Part model, mm, in its own coordinate system. Round coordinates to 2 decimals unless told otherwise and drop trailing zeros. Loops run counter-clockwise (first coordinate to the right, second up) from the corner with the lowest first, then second, coordinate; pieces in that order, holes last.
(1) Mould opens along X. For faces 1 (the face through (-27.1, 3.04, 51.66)), 2 (the face through (28.9, 3.04, 51.66)), 3 (the face through (-1, 6, -2)), 4 (the face through (85, 3, 2)) say: +X half, -X half, draft (parallel to the pull), parting line (faces both ways), or undercut.
(2) Cut at C-C on x = -42.5. List the corners of the cut face in (y, z).
(3) Cut at B-B on y = 4. Count the separate pieces of the cut face and the enclosed holes in it, then the cut area to 3 significant figures.
(4) Flat gauge pin, fed straight in: pin 1 (8 mm diameter, centred on x = 0, z = -13.7, fed in from +Y). Where does the tip first touch, or does it go through?
(5) Probe probe 1 along X at (y, z) = (3.3, 48.8); probe 2 along X at (y, z) = (4, 92.5); probe 3 along X at (y, z) = (3.5, -124.5). List the from-to ranges inside material, lowest first.
(6) Cut at D-D on z = -13.7. List the corners of the cut face in (x, y), then the cut area to 3 significant figures.
(7) Cut at A-A on z = 92.5. List the corners of the cut face in (x, y).
from build123d import *

# Parameters (mm, degrees)
SKETCH1_W           = 170
SKETCH1_H           = 280
BOSS_EXTRUDE1_DEPTH = 6
SKETCH2_R           = 5
CUT_EXTRUDE1_DEPTH  = 6
SKETCH4_R           = 22.5
SKETCH4_R_2         = 3
CUT_EXTRUDE3_DEPTH  = 10


with BuildPart() as part:
    # Sketch1 → Boss-Extrude1 (new body)
    with BuildSketch(Plane(origin=(0, 0, 0), x_dir=(1, 0, 0), z_dir=(0, 1, 0))):
        Rectangle(SKETCH1_W, SKETCH1_H)
    extrude(amount=BOSS_EXTRUDE1_DEPTH)

    # Sketch2 → Cut-Extrude1 (cut)
    with BuildSketch(Plane(origin=(0, 6, 0), x_dir=(1, 0, 0), z_dir=(0, 1, 0))):
        with Locations(Location((-57.5, 120, 0), (0, 0, 270))):
            Circle(SKETCH2_R)
        with Locations(Location((57.5, 120, 0), (0, 0, 270))):
            Circle(SKETCH2_R)
        with Locations(Location((0, 13.7, 0), (0, 0, 270))):
            Circle(SKETCH2_R)
        with Locations(Location((-57.5, -120, 0), (0, 0, 270))):
            Circle(SKETCH2_R)
        with Locations(Location((57.5, -120, 0), (0, 0, 270))):
            Circle(SKETCH2_R)
        with Locations(Location((-42.5, -92.5, 0), (0, 0, 270))):
            Circle(SKETCH2_R)
        with Locations(Location((42.5, -92.5, 0), (0, 0, 270))):
            Circle(SKETCH2_R)
    extrude(amount=-CUT_EXTRUDE1_DEPTH, mode=Mode.SUBTRACT)

    # Sketch4 → Cut-Extrude3 (cut)
    with BuildSketch(Plane(origin=(0, 6, 0), x_dir=(1, 0, 0), z_dir=(0, 1, 0))):
        with Locations(Location((0, -48.8, 0), (0, 0, 270))):
            Circle(SKETCH4_R)
        with Locations(Location((28, -48.8, 0), (0, 0, 270))):
            Circle(SKETCH4_R_2)
        with Locations(Location((-28, -48.8, 0), (0, 0, 270))):
            Circle(SKETCH4_R_2)
    extrude(amount=-CUT_EXTRUDE3_DEPTH, mode=Mode.SUBTRACT)


solid = part.part
Final values:
1. face 1: undercut
1. face 2: undercut
1. face 3: draft
1. face 4: +X half
2. outline: (0, -140) - (6, -140) - (6, 87.5) - (0, 87.5) - close; (0, 97.5) - (6, 97.5) - (6, 140) - (0, 140) - close
3. separate pieces: 1
3. enclosed holes: 10
3. area: 45,400 mm2
4. pin 1: passes through
5. probe 1: x = -85 to -31, -25 to -22.5, 22.5 to 25, 31 to 85
5. probe 2: x = -85 to -47.5, -37.5 to 37.5, 47.5 to 85
5. probe 3: x = -85 to -59.68, -55.32 to 55.32, 59.68 to 85
6. outline: (-85, 0) - (-5, 0) - (-5, 6) - (-85, 6) - close; (5, 0) - (85, 0) - (85, 6) - (5, 6) - close
6. area: 960 mm2
7. outline: (-85, 0) - (-47.5, 0) - (-47.5, 6) - (-85, 6) - close; (-37.5, 0) - (37.5, 0) - (37.5, 6) - (-37.5, 6) - close; (47.5, 0) - (85, 0) - (85, 6) - (47.5, 6) - close
